Geometry: final body of the model. Coordinates: model frame, mm. A direction names the side the tool comes from. Give positions to 0.01 mm unless a question says otherwise; leave off trailing zeros. Order: outer loops, then holes, each group sorted by start corner. A loop starts at its lowest first (then second) coordinate and runs counter-clockwise, first axis right, second up. Notation, with made-up numbers: M 80.25,-2.75 L 90.25,-2.75 A13 ccw 90.25,17.25 Z; hole C -22,55 d8. An arc over 180 degrees is marked long. Use CSV: the item, a comma, the result in double quotes.
```python
from build123d import *

# Parameters (mm, degrees)
SKETCH4_W           = 31.05
SKETCH4_H           = 19.05
BOSS_EXTRUDE1_DEPTH = 19
SHELL1_T            = 2
SKETCH5_W           = 12
SKETCH5_H           = 19.05
CUT_EXTRUDE1_DEPTH  = 2


with BuildPart() as part:
    # Sketch4 → Boss-Extrude1 (new body)
    with BuildSketch(Plane(origin=(0, 0, 0), x_dir=(0, 0, -1), z_dir=(1, 0, 0))):
        Rectangle(SKETCH4_W, SKETCH4_H)
    extrude(amount=BOSS_EXTRUDE1_DEPTH)

    # Shell1
    shell1_openings = [part.faces().sort_by_distance(p)[0] for p in [
        (0, 0, 0),
    ]]
    offset(amount=SHELL1_T, openings=shell1_openings, kind=Kind.INTERSECTION)

    # Sketch5 → Cut-Extrude1 (cut)
    with BuildSketch(Plane(origin=(0, 0, -17.525), x_dir=(-1, 0, 0), z_dir=(0, 0, -1))):
        with Locations((-6, 0)):
            Rectangle(SKETCH5_W, SKETCH5_H)
    extrude(amount=-CUT_EXTRUDE1_DEPTH, mode=Mode.SUBTRACT)


solid = part.part
```
1. Section C-C, the plane x = 2.5. Return the cut outline in (y, z) (3 decimals), plus the area to 3 significant figures.
Answer:
outline,"M -11.525,-17.525 L -9.525,-17.525 L -9.525,15.525 L 9.525,15.525 L 9.525,-17.525 L 11.525,-17.525 L 11.525,17.525 L -11.525,17.525 Z"
area,"178 mm2"
2. Reachability of faces 1 (the face through (10, -11.525, 0)), 2 (the face through (12, 0, -17)), 3 (the face through (15, 0, -15.525)) from +Z, -Z, +X, -X, +Y, -Y: full face, straight path, thin tool, end or side. Return the list, or none.
Answer:
face 1,"+Z, -Z, +X, -X, -Y"
face 2,"-Z, -X"
face 3,"-X"
3. Pull-direction query (Z, two-part tool) for faces 4 (the face through (9, 9.525, -1)), 5 (the face through (15, 0, -17.525)), 6 (the face through (10, 11.525, 0)); classes: +Z half, -Z half, draft (parallel to the pull), parting line (faces both ways), or undercut.
Answer:
face 4,"undercut"
face 5,"-Z half"
face 6,"draft"
4. Pin query (flat end, axial travel): pin 1 Ø4 at (y, z) = (-3.5, 11) entering from -X; pin 2 Ø0.6 at (y, z) = (-0.5, -16) entering from -X. Return the tip coordinate at first contact, or that it passes through.
Answer:
pin 1,"x = 19"
pin 2,"x = 12"
5. Line query: line 1 (Z direction, x = 17.25, y = -4) (3 decimals); line 2 (Y direction, x = 7.25, z = -2) (3 decimals); line 3 (X direction, y = -8, z = -5). Output: solid intervals per line, ascending.
Answer:
line 1,"-17.525 to -15.525, 15.525 to 17.525"
line 2,"-11.525 to -9.525, 9.525 to 11.525"
line 3,"19 to 21"
6. Section A-A, the plane x = 13.25. Return the cut outline in (y, z) (3 decimals).
Answer:
outline,"M -11.525,-17.525 L 11.525,-17.525 L 11.525,17.525 L -11.525,17.525 Z; hole M -9.525,-15.525 L 9.525,-15.525 L 9.525,15.525 L -9.525,15.525 Z"
7. Section B-B, the plane y = -8. Return the cut outline in (x, z) (3 decimals), plus the area to 3 significant figures.
Answer:
outline,"M 0,15.525 L 19,15.525 L 19,-15.525 L 12,-15.525 L 12,-17.525 L 21,-17.525 L 21,17.525 L 0,17.525 Z"
area,"122 mm2"
